The listing builds one solid part. Answer for the finished solid, in the listing's coordinates (mm). Face numbers are marked on the shaded views. Coordinates: 2 decimals unless noted, no trailing zeros. Write each loop counter-clockwise with the first axis right and the second up, starting at its lowest first coordinate (ties: lowest second). Pieces come first, ordered by that corner, then holes.
(1) The part is cut by section A-A on z = 28. Determine the outline of the cut face in (x, y), plus the area to 3 significant figures.
(2) The part is cut by section B-B on x = 0. Determine the outline of the cut face in (y, z), plus the area to 3 significant figures.
(3) Given P1, Ø6, axis at x = 11.5, z = 41.5, coming from the -Y side; P2, Ø7.5, axis at x = 1.5, y = 1.5, coming from the +Z side, each flat-ended and moving along its own axis, determine where each tip first touches the part or whether it passes through.
(4) For a pull along X with two mould halves and no side action, classify the marked faces 1, 2 and 3 as +X half, -X half, draft (parallel to the pull), parting line (faces both ways), or undercut.
(5) The part is cut by section D-D on z = 7. Determine the outline of the cut face in (x, y), plus the area to 3 significant figures.
(6) Straight lines are drawn through the part: line 1 (Y direction, x = 0, z = 51); line 2 (Z direction, x = 3.5, y = -4.25); line 3 (X direction, y = -6.5, z = 39.5). For each, find the intervals that lie inside material, in ascending order.
from build123d import *

# Parameters (mm, degrees)
F1_R     = 15
F2_DEPTH = 67.678692
F3_T     = -2.5
F0_R     = 15
F4_DEPTH = 25


with BuildPart() as f2:
    # F1 (on face) → F2 (new body)
    with BuildSketch(Plane.XY):
        Circle(F1_R)
    extrude(amount=F2_DEPTH)

    # F3
    f3_openings = [f2.faces().sort_by_distance(p)[0] for p in [
        (0, 0, 67.678692),
    ]]
    offset(amount=F3_T, openings=f3_openings)

    # F0 (on Top) → F4 (join)
    with BuildSketch(Plane.XY):
        Circle(F0_R)
    extrude(amount=F4_DEPTH)


solid = f2.part
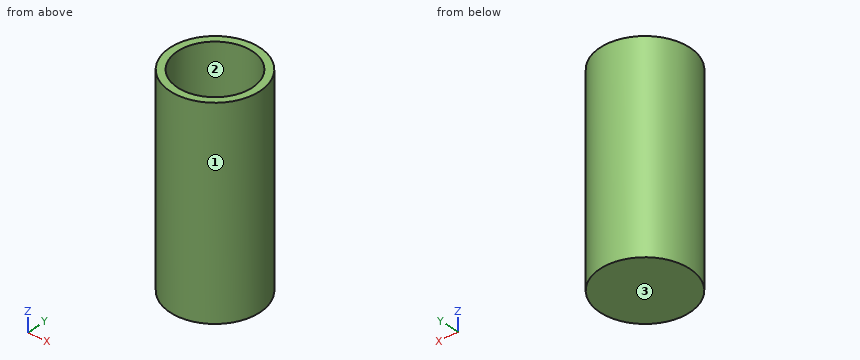
Model answer:
1. outline: circle Ø30 at (0, 0); hole circle Ø25 at (0, 0)
1. area: 216 mm2
2. outline: (-15, 0) - (15, 0) - (15, 67.68) - (12.5, 67.68) - (12.5, 25) - (-12.5, 25) - (-12.5, 67.68) - (-15, 67.68) - close
2. area: 963 mm2
3. P1: stops at y = -12.36
3. P2: stops at z = 25
4. face 1: parting line
4. face 2: undercut
4. face 3: draft
5. outline: circle Ø30 at (0, 0)
5. area: 707 mm2
6. line 1: y = -15 to -12.5, 12.5 to 15
6. line 2: z = 0 to 25
6. line 3: x = -13.52 to -10.68, 10.68 to 13.52
